Could you check a few things on this model? Use its own coordinates, in mm. Face numbers are marked on the shaded views. A direction names the side the tool comes from. Give positions to 0.01 mm unless a question says otherwise; leave off trailing zeros. Loops run counter-clockwise (first coordinate to the right, second up) from the corner with the lowest first, then second, coordinate; pieces in that order, holes last. Notation, with made-up numbers: (-39.75, -20) - (-28.75, -20) arc R23 ccw to (-28.75, -4) - close; hole circle Ø1 at (82.25, -6). An arc over 180 degrees is marked (long way). Write each question's results on one line, items separated by ' | '. Start each with the question number.
(1) For pin 1 (2 mm diameter, centred on x = -10.94, y = 15.83, fed in from -Z); pin 2 (4 mm diameter, centred on x = -5.5, y = 3.5, fed in from +Z); pin 3 (1.5 mm diameter, centred on y = 8.5, z = -0.5, fed in from -X), each with a flat end and sliding along its axis, tell me the tip position at first contact or that it passes through.
(2) If we mould it in two halves opening along Y, with no side actions, what happens to the marked faces 1, 2 and 3? For each: released by +Y, released by -Y, zero draft, split by the parting line, or undercut.
(3) Suppose I cut it at D-D (z = -2.3). Please give me the cut outline in (x, y).
(4) On a 3-axis mill with a long thin cutter (end or side, diameter ignored), from which of +Z, -Z, +X, -X, +Y, -Y can I reach the whole of each face in a straight line? I mean the marked faces 4 and 5. Say none if no direction works.
(5) Suppose I cut it at C-C (x = 0). Please give me the cut outline in (y, z), and give its area (3 significant figures).
(6) Suppose I cut it at A-A (y = 0). Please give me the cut outline in (x, z), and give its area (3 significant figures).
(7) I need wall thicknesses on line 1 (Y direction, x = -12, z = -1.4); line 2 (Y direction, x = -7.25, z = -1.4); line 3 (Y direction, x = -5.5, z = -1.2). Which ranges of each line are inside material? Lowest first, please.
(8) Suppose I cut it at B-B (z = -0.65). Please give me the cut outline in (x, y).
Autodesk Inventor part; units mm, degrees
ref_plane "YZ Plane" through (0, 0, 0) normal (1, 0, 0) x (0, 1, 0)
ref_plane "XZ Plane" through (0, 0, 0) normal (0, 1, 0) x (-1, 0, 0)
ref_plane "XY Plane" through (0, 0, 0) normal (0, 0, 1) x (1, 0, 0)
sketch "Sketch2" plane through (0, 0, 0) normal (0, 0, 1) x (1, 0, 0)
  line L0 (0, 0) -> (-12.7279, 12.7279) construction
  line L1 (0, 0) -> (18, 0) construction
  line L2 (0, 0) -> (-12.7279, 12.7279) construction
  line L3 (-3.5355, -3.5355) -> (-16.2635, 9.1924) construction
  line L4 (-9.1924, 16.2635) -> (3.5355, 3.5355) construction
  arc A0 (-3.5355, -3.5355) -> (-1.5844, -4.7423) centre (0, 0) ccw construction
  arc A1 (-9.1924, 16.2635) -> (-16.2635, 9.1924) centre (-12.7279, 12.7279) ccw
  arc A2 (-6.5476, 19.2704) -> (-19.2704, 6.5476) centre (-12.7279, 12.7279) ccw
  arc A3 (-19.2704, 6.5476) -> (-1.5844, -4.7423) centre (12.0821, 36.1644) ccw
  arc A4 (4.7423, 1.5844) -> (-6.5476, 19.2704) centre (-36.1644, -12.0821) ccw
  arc A5 (-3.9009, 10.972) -> (-6.5476, 19.2704) centre (-12.7279, 12.7279) ccw construction
  arc A6 (-6.364, 6.364) -> (-3.9009, 10.972) centre (-12.7279, 12.7279) ccw construction
  arc A7 (-10.972, 3.9009) -> (-6.364, 6.364) centre (-12.7279, 12.7279) ccw construction
  arc A8 (-19.2704, 6.5476) -> (-10.972, 3.9009) centre (-12.7279, 12.7279) ccw construction
  arc A9 (4.7423, 1.5844) -> (3.5355, 3.5355) centre (0, 0) ccw construction
  circle A10 centre (0, 0) radius 5
  circle A11 centre (0, 0) radius 3.025 construction
  circle A12 centre (0, 0) radius 1.25
  line L5 (0, 0) -> (-12.7279, 12.7279) construction
  line L6 (0, 0) -> (18, 0) construction
  line L7 (0, 0) -> (-12.7279, 12.7279) construction
  line L8 (-3.5355, -3.5355) -> (-16.2635, 9.1924) construction
  line L9 (-9.1924, 16.2635) -> (3.5355, 3.5355) construction
  arc A13 (-3.5355, -3.5355) -> (-1.5844, -4.7423) centre (0, 0) ccw construction
  arc A14 (-9.1924, 16.2635) -> (-16.2635, 9.1924) centre (-12.7279, 12.7279) ccw
  arc A15 (-6.5476, 19.2704) -> (-19.2704, 6.5476) centre (-12.7279, 12.7279) ccw
  circle A16 centre (-10.9381, 15.8279) radius 1.25
  circle A17 centre (-10.9381, 15.8279) radius 3.1 construction
  circle A18 centre (-16.3075, 12.7279) radius 1.25
  circle A19 centre (-16.3075, 12.7279) radius 3.1 construction
  circle A20 centre (-10.9381, 9.6279) radius 1.25
  circle A21 centre (-10.9381, 9.6279) radius 3.1 construction
  arc A22 (-19.2704, 6.5476) -> (-1.5844, -4.7423) centre (12.0821, 36.1644) ccw
  arc A23 (4.7423, 1.5844) -> (-6.5476, 19.2704) centre (-36.1644, -12.0821) ccw
  arc A24 (-3.9009, 10.972) -> (-6.5476, 19.2704) centre (-12.7279, 12.7279) ccw construction
  arc A25 (-6.364, 6.364) -> (-3.9009, 10.972) centre (-12.7279, 12.7279) ccw construction
  arc A26 (-10.972, 3.9009) -> (-6.364, 6.364) centre (-12.7279, 12.7279) ccw construction
  arc A27 (-19.2704, 6.5476) -> (-10.972, 3.9009) centre (-12.7279, 12.7279) ccw construction
  arc A28 (4.7423, 1.5844) -> (3.5355, 3.5355) centre (0, 0) ccw construction
  circle A29 centre (0, 0) radius 5
  circle A30 centre (0, 0) radius 3.025 construction
  circle A31 centre (0, 0) radius 1.25
  point P0 (-6.364, 6.364)
  point P1 (-11.1244, -0.1893)
  point P2 (-6.364, 6.364)
  point P3 (-11.1244, -0.1893)
  point P4 (4.7423, 1.5844)
  point P5 (-1.5844, -4.7423)
  dimension "d47" = 18
  dimension "d48" = 135
  dimension "d49" = 5
  dimension "d50" = 18
  dimension "d54" = 8
  dimension "d55" = 10
  dimension "d56" = 6.05
  dimension "d57" = 2.5
  dimension "d58" = 18
  dimension "d59" = 135
  dimension "d60" = 5
  dimension "d61" = 18
  dimension "d62" = 2.5
  dimension "d63" = 6.2
  dimension "d64" = 360
  dimension "d65" = 8
  dimension "d66" = 10
  dimension "d67" = 6.05
  dimension "d68" = 2.5
extrude "Extrusion2" add sketch "Sketch2" against normal blind 3
chamfer "Chamfer3" distance 1.75 angle 45 3 edges at (-12.1881, 15.8279, 0) (-17.5575, 12.7279, 0) (-12.1881, 9.6279, 0)
sketch "Sketch3" plane through (0, 0, 0) normal (0, 0, 1) x (1, 0, 0)
  circle A0 centre (-10.9381, 9.6279) radius 3
  arc A1 (-19.2704, 6.5476) -> (-1.5844, -4.7423) centre (12.0821, 36.1644) ccw
  circle A2 centre (0, 0) radius 1.25
  arc A3 (4.7423, 1.5844) -> (-6.5476, 19.2704) centre (-36.1644, -12.0821) ccw
  circle A4 centre (-16.3075, 12.7279) radius 3
  circle A5 centre (-10.9381, 15.8279) radius 3
  arc A6 (-1.5757, 8.2644) -> (-5.2092, 7.8448) centre (-3.2996, 7.2504) ccw
  arc A7 (-7.6726, 4.5944) -> (-7.5631, 1.1727) centre (-6.584, 2.9166) ccw
  arc A8 (-7.6726, 4.5944) -> (-5.2092, 7.8448) centre (-10.9381, 9.6279) ccw
  arc A9 (-7.5631, 1.1727) -> (-6.6808, 0.6917) centre (12.0821, 36.1644) ccw
  arc A10 (-0.6917, 6.6808) -> (-1.5757, 8.2644) centre (-36.1644, -12.0821) ccw
  arc A11 (-6.6808, 0.6917) -> (-3.9071, 1.6726) centre (-5.7457, 2.4596) ccw
  arc A12 (-1.6726, 3.9071) -> (-0.6917, 6.6808) centre (-2.4596, 5.7457) ccw
  arc A13 (-1.6726, 3.9071) -> (-3.9071, 1.6726) centre (0, 0) ccw
  dimension "d77" = 3
  dimension "d78" = 2
  dimension "d79" = 2
  dimension "d80" = 3
  dimension "d81" = 3
  dimension "d82" = 2
  dimension "d83" = 2
  dimension "d84" = 3
extrude "Extrusion3" cut sketch "Sketch3" against normal blind 1.5 contours A10 A12 A13 A11 A9 A7 A8 A6
properties part number "クランク_前" material "Aluminum 2014-T6"
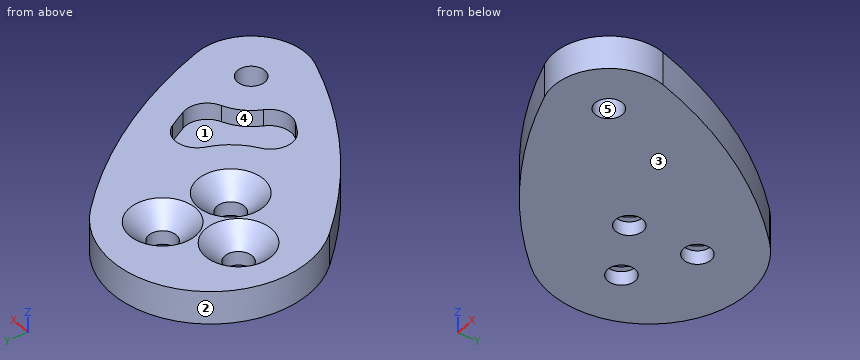
Output values:
1) pin 1: through | pin 2: z = -1.5 | pin 3: x = -21.03
2) face 1: undercut | face 2: split by the parting line | face 3: zero draft
3) outline: (-19.27, 6.55) arc R43.13 ccw to (-1.58, -4.74) arc R5 ccw to (4.74, 1.58) arc R43.13 ccw to (-6.55, 19.27) arc R9 ccw to start; hole circle Ø2.5 at (-16.31, 12.73); hole circle Ø2.5 at (-10.94, 9.63); hole circle Ø2.5 at (-10.94, 15.83); hole circle Ø2.5 at (0, 0)
4) face 4: +Z | face 5: +Z, -Z
5) outline: (-5, -3) - (-1.25, -3) - (-1.25, 0) - (-5, 0) - close; (1.25, -3) - (11.42, -3) - (11.42, 0) - (1.25, 0) - close | area: 41.8 mm2
6) outline: (-11.42, -3) - (-1.25, -3) - (-1.25, 0) - (-11.42, 0) - close; (1.25, -3) - (5, -3) - (5, 0) - (1.25, 0) - close | area: 41.8 mm2
7) line 1: 0.38 to 8.43, 10.82 to 14.63, 17.02 to 21.7 | line 2: -2.39 to 1, 4.9 to 19.87 | line 3: -3.22 to 0.47, 7.09 to 18.25
8) outline: (-19.27, 6.55) arc R43.13 ccw to (-1.58, -4.74) arc R5 ccw to (4.74, 1.58) arc R43.13 ccw to (-6.55, 19.27) arc R9 ccw to start; hole circle Ø4.7 at (-16.31, 12.73); hole circle Ø4.7 at (-10.94, 9.63); hole circle Ø4.7 at (-10.94, 15.83); hole (-7.67, 4.59) arc R2 ccw to (-7.56, 1.17) arc R40.6 ccw to (-6.68, 0.69) arc R2 ccw to (-3.91, 1.67) arc R4.25 cw to (-1.67, 3.91) arc R2 ccw to (-0.69, 6.68) arc R40.11 ccw to (-1.58, 8.26) arc R2 ccw to (-5.21, 7.84) arc R6 cw to start; hole circle Ø2.5 at (0, 0)
